Source: CAD feature listing. Evaluate the final solid. Frame: model axes, mm. Face numbers are marked on the shaded views. Give positions to 0.01 mm unless a question says otherwise; leave off trailing zeros. Loops run counter-clockwise (first coordinate to the right, second up) from the corner with the lowest first, then second, coordinate; pieces in that order, holes last. Notation, with made-up numbers: (76, 20.5) -> (121, 20.5) arc R27 ccw to (121, 49.5) -> close; hole circle Ø7 at (-33, 41). An arc over 180 degrees is marked (long way). Return JSON: item names as keys, results as strings. Group by question number.
(1) Cut plane D-D on x = -9. Return loops of the section in (y, z).
(2) Cut plane A-A on y = 19.5. Return loops of the section in (x, z).
(3) Pin query (flat end, axial travel): pin 1 (1 mm diameter, centred on x = 120, z = -7, fed in from -Y); pin 2 (10 mm diameter, centred on y = -17.5, z = 28.5, fed in from +X); pin 3 (10 mm diameter, centred on x = 3, z = 19, fed in from +Y). Return the tip coordinate at first contact, or that it passes through.
(4) Ray query, line 1 (Z direction, x = -9.5, y = 21.5); line 2 (Z direction, x = -55.5, y = 16); line 3 (X direction, y = 20.5, z = 49). Return the intervals inside material, ascending. Write a range as from..to.
(5) Cut plane B-B on z = 26.5. Return loops of the section in (x, y), then the cut area to 3 significant figures.
(6) Draft query along X for the marked faces 1, 2 and 3. Return one class per face: released by +X, released by -X, zero draft, split by the parting line, or undercut.
(7) Cut plane C-C on y = -16. Return loops of the section in (x, z), then the cut area to 3 significant figures.
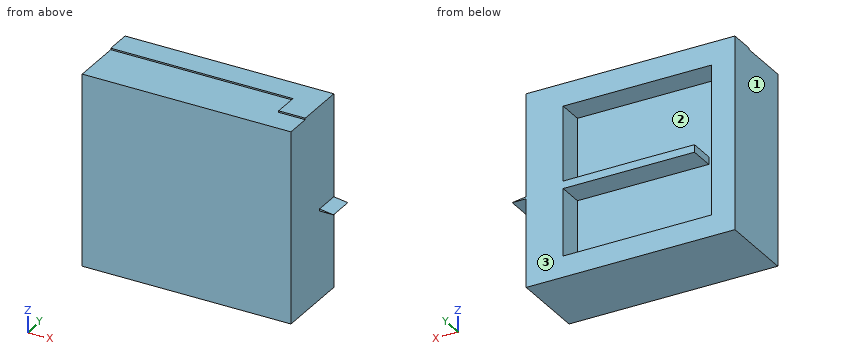
```python
from build123d import *

# Parameters (mm, degrees)
F0_W      = 193.780676
F0_H      = 193.357542
F1_DEPTH  = 25.4
F2_W      = 185.913056
F2_H      = 193.357542
F3_DEPTH  = 25.4
F4_W      = 25.4
F4_H      = 193.357542
F5_DEPTH  = 25.4
F6_W      = 26.91965
F6_H      = 194.875538
F7_DEPTH  = 25.4
F8_W      = 211.313056
F8_H      = 194.875538
F8_W_2    = 150.167435
F8_H_2    = 150.83959
F9_DEPTH  = 25.4
F11_DEPTH = 25.4


with BuildPart() as f1:
    # F0 (on Front) → F1 (new body)
    with BuildSketch(Plane.XZ):
        with Locations((-0.897467, -0.267394)):
            Rectangle(F0_W, F0_H)
    extrude(amount=F1_DEPTH)

    # F2 (on face) → F3 (join)
    with BuildSketch(Plane.XZ.offset(25.4)):
        with Locations((-4.831277, -0.267394)):
            Rectangle(F2_W, F2_H)
    extrude(amount=F3_DEPTH)

    # F4 (on face) → F5 (join)
    with BuildSketch(Plane.YZ.offset(88.125251)):
        with Locations((-38.1, -0.267394)):
            Rectangle(F4_W, F4_H)
    extrude(amount=F5_DEPTH)

    # F6 (on face) → F7 (join)
    with BuildSketch(Plane(origin=(0, -25.4, 0), x_dir=(-1, 0, 0), z_dir=(0, 1, 0))):
        with Locations((-100.065426, 0.491604)):
            Rectangle(F6_W, F6_H)
    extrude(amount=F7_DEPTH)

    # F8 (on face) → F9 (join)
    with BuildSketch(Plane(origin=(0, 0, 0), x_dir=(-1, 0, 0), z_dir=(0, 1, 0))):
        with Locations((-7.868723, 0.491604)):
            Rectangle(F8_W, F8_H)
        with Locations((-0.97549, -0.210028)):
            Rectangle(F8_W_2, F8_H_2, mode=Mode.SUBTRACT)
    extrude(amount=F9_DEPTH)

    # F10 (on face) → F11 (join)
    with BuildSketch(Plane(origin=(0, 0, 0), x_dir=(-1, 0, 0), z_dir=(0, 1, 0))):
        Polygon((56.883931, -0.210028), (0, 0), (-76.059207, -0.210028), (-127.674758, -7.74778), (56.8561, -7.74778), align=None)
    extrude(amount=F11_DEPTH)


solid = f1.part
```
Answers:
{
 "1": {"outline": "(-50.8, -96.95) -> (25.4, -96.95) -> (25.4, -75.63) -> (0, -75.63) -> (0, -7.75) -> (25.4, -7.75) -> (25.4, -0.03) -> (0, -0.03) -> (0, 75.21) -> (25.4, 75.21) -> (25.4, 97.93) -> (0, 97.93) -> (0, 96.41) -> (-50.8, 96.41) -> close"},
 "2": {"outline": "(-97.79, -96.95) -> (113.53, -96.95) -> (113.53, -7.75) -> (127.67, -7.75) -> (113.53, -5.68) -> (113.53, 97.93) -> (-97.79, 97.93) -> close; hole (-74.11, -75.63) -> (76.06, -75.63) -> (76.06, -7.75) -> (-56.86, -7.75) -> (-56.88, -0.21) -> (0, 0) -> (76.06, -0.21) -> (76.06, 75.21) -> (-74.11, 75.21) -> close"},
 "3": {"pin 1": "y = 0", "pin 2": "x = 113.53", "pin 3": "y = 0"},
 "4": {"line 1": "-96.95..-75.63, -7.75..-0.04, 75.21..97.93", "line 2": "-96.95..-75.63, -7.75..-0.2, 75.21..97.93", "line 3": "-97.79..-74.11, 76.06..113.53"},
 "5": {"outline": "(-97.79, -50.8) -> (113.53, -50.8) -> (113.53, 25.4) -> (76.06, 25.4) -> (76.06, 0) -> (-74.11, 0) -> (-74.11, 25.4) -> (-97.79, 25.4) -> close", "area": "12,300 mm²"},
 "6": {"face 1": "released by -X", "face 2": "undercut", "face 3": "zero draft"},
 "7": {"outline": "(-97.79, -96.95) -> (113.53, -96.95) -> (113.53, 97.93) -> (86.61, 97.93) -> (86.61, 96.41) -> (-97.79, 96.41) -> close", "area": "40,900 mm²"}
}
